```python
from build123d import *

# Parameters (mm, degrees)
BOSS_EXTRU_1_DEPTH      = 7.62
ESQUISSE3_W             = 0.8
ESQUISSE3_H             = 1.27
ENL_V_MAT_EXTRU_1_DEPTH = 8.9
ESQUISSE4_W             = 2.4
ESQUISSE4_H             = 0.5
ENL_V_MAT_EXTRU_2_DEPTH = 8.62
ESQUISSE2_W             = 0.6
ESQUISSE2_H             = 0.6
BOSS_EXTRU_2_DEPTH      = 3.5
BOSS_EXTRU_2_DEPTH_BACK = 9
BOSS_EXTRU_3_DEPTH      = 5.08
CHANFREIN4_SIZE         = 0.15
CHANFREIN5_SIZE         = 0.4


with BuildPart() as part:
    # Esquisse1 → Boss.-Extru.1 (new body)
    with BuildSketch(Plane.XY):
        Polygon((0, 11.4), (0, 0), (5, 0), (5, 11.4), (4.2, 11.4), (4.2, 2.5), (0.8, 2.5), (0.8, 11.4), align=None)
    extrude(amount=BOSS_EXTRU_1_DEPTH)

    # Esquisse3 → Enlèv. mat.-Extru.1 (cut)
    with BuildSketch(Plane(origin=(0, 11.4, 0), x_dir=(1, 0, 0), z_dir=(0, 1, 0))):
        with Locations((0.4, -0.635)):
            Rectangle(ESQUISSE3_W, ESQUISSE3_H)
        with Locations((0.4, -6.985)):
            Rectangle(ESQUISSE3_W, ESQUISSE3_H)
    extrude(amount=-ENL_V_MAT_EXTRU_1_DEPTH, mode=Mode.SUBTRACT)

    # Esquisse4 → Enlèv. mat.-Extru.2 (cut, through all)
    with BuildSketch(Plane.XY.offset(7.62)):
        with Locations((2.5, 0.25)):
            Rectangle(ESQUISSE4_W, ESQUISSE4_H)
    extrude(amount=-ENL_V_MAT_EXTRU_2_DEPTH, mode=Mode.SUBTRACT)

    # Esquisse2 → Boss.-Extru.2 (add, two sides)
    with BuildSketch(Plane.XZ.offset(-0.5)) as boss_extru_2_sk:
        with Locations((2.5, 6.35)):
            Rectangle(ESQUISSE2_W, ESQUISSE2_H)
        with Locations((2.5, 1.27)):
            Rectangle(ESQUISSE2_W, ESQUISSE2_H)
        with Locations((2.5, 3.81)):
            Rectangle(ESQUISSE2_W, ESQUISSE2_H)
    extrude(amount=BOSS_EXTRU_2_DEPTH)
    extrude(boss_extru_2_sk.sketch, amount=-BOSS_EXTRU_2_DEPTH_BACK)

    # Esquisse5 → Boss.-Extru.3 (add)
    with BuildSketch(Plane.XY.offset(6.35)):
        Polygon((0.8, 9.5), (1.2, 8.5), (0.8, 8.5), align=None)
    extrude(amount=-BOSS_EXTRU_3_DEPTH)

    # Chanfrein4
    chanfrein4_edges = [part.edges().sort_by_distance(p)[0] for p in [
        (2.8, 9.5, 3.81),
        (2.5, 9.5, 3.51),
        (2.2, 9.5, 3.81),
        (2.5, 9.5, 4.11),
        (2.8, -3, 3.81),
        (2.5, -3, 4.11),
        (2.2, -3, 3.81),
        (2.5, -3, 3.51),
        (2.8, 9.5, 6.35),
        (2.5, 9.5, 6.05),
        (2.2, 9.5, 6.35),
        (2.5, 9.5, 6.65),
        (2.8, -3, 6.35),
        (2.5, -3, 6.65),
        (2.2, -3, 6.35),
        (2.5, -3, 6.05),
        (2.8, 9.5, 1.27),
        (2.5, 9.5, 0.97),
        (2.2, 9.5, 1.27),
        (2.5, 9.5, 1.57),
        (2.8, -3, 1.27),
        (2.5, -3, 1.57),
        (2.2, -3, 1.27),
        (2.5, -3, 0.97),
    ]]
    chamfer(chanfrein4_edges, length=CHANFREIN4_SIZE)

    # Chanfrein5
    chanfrein5_edges = [part.edges().sort_by_distance(p)[0] for p in [
        (4.2, 11.4, 3.81),
        (0.8, 11.4, 3.81),
    ]]
    chamfer(chanfrein5_edges, length=CHANFREIN5_SIZE)


solid = part.part
```
The model under review builds one solid part; all positions refer to its coordinate system, in mm. A direction names the side the tool comes from. Round coordinates to 2 decimals unless told otherwise and drop trailing zeros. Order: outer loops, then holes, each group sorted by start corner. A loop starts at its lowest first (then second) coordinate and runs counter-clockwise, first axis right, second up. Notation, with made-up numbers: (7, 50) -> (66, 50) arc R19 ccw to (66, 87) -> close; hole circle Ø9 at (30.5, 66.5). An arc over 180 degrees is marked (long way). One line per item, written item: value. Start each with the question number.
Q1. Take a section at C-C (z = 4.5). Write out the cut boundary in (x, y), and give its area (3 significant figures).
Q2. Mouldability with a two-part tool opening along Y and no side actions: class faces 4 (the face through (1, 0, 4)), 5 (the face through (3, 2, 0)), 6 (the face through (1, 9, 4)), 7 (the face through (0.8, 5, 4)) as released by +Y, released by -Y, zero draft, split by the parting line, or undercut.
Q3. Machinability: for faces 1 (the face through (4, 0, 4)), 2 (the face through (0.5, 7, 6.35)), 3 (the face through (0.8, 10, 4)), which of the approach directions +Z, -Z, +X, -X, +Y, -Y give a long, thin tool a straight path to every point of the face, cutting with its end or side? Answer none if there is none.
Q4. Take a section at A-A (y = -0.25). Write out the cut boundary in (x, z).
Q5. Clearance check with flat-ended pins moving along their axes: pin 1 Ø1 at (x, y) = (2.5, 6.5) entering from -Z; pin 2 Ø0.5 at (y, z) = (-1.5, 4) entering from -X; pin 3 Ø2 at (x, y) = (1, 9) entering from -Z. State where each tip first meets the part, or that it passes through.
Q6. Take a section at B-B (y = 8). Write out the cut boundary in (x, z).
Q7. Wall thickness on line 1 (Z direction, x = 2.7, y = 6.75); line 2 (X direction, y = 7.25, z = 6); line 3 (X direction, y = 6.5, z = 0.5): over which ranges is each line inside the solid? List them lowest first.
Q8. Take a section at D-D (x = 1.85). Write out the cut boundary in (y, z).
Reported:
1. outline: (0, 0) -> (1.3, 0) -> (1.3, 0.5) -> (3.7, 0.5) -> (3.7, 0) -> (5, 0) -> (5, 11.4) -> (4.6, 11.4) -> (4.2, 11) -> (4.2, 2.5) -> (0.8, 2.5) -> (0.8, 8.5) -> (1.2, 8.5) -> (0.8, 9.5) -> (0.8, 11) -> (0.4, 11.4) -> (0, 11.4) -> close
1. area: 25.6 mm2
2. face 4: released by -Y
2. face 5: zero draft
2. face 6: released by +Y
2. face 7: undercut
3. face 1: +Z, -Z, +X, -Y
3. face 2: +Z, -X, +Y
3. face 3: +Z, -Z, +Y
4. outline: (2.2, 0.97) -> (2.8, 0.97) -> (2.8, 1.57) -> (2.2, 1.57) -> close; (2.2, 3.51) -> (2.8, 3.51) -> (2.8, 4.11) -> (2.2, 4.11) -> close; (2.2, 6.05) -> (2.8, 6.05) -> (2.8, 6.65) -> (2.2, 6.65) -> close
5. pin 1: stops at z = 0.97
5. pin 2: stops at x = 2.2
5. pin 3: stops at z = 1.27
6. outline: (0, 1.27) -> (0.8, 1.27) -> (0.8, 6.35) -> (0, 6.35) -> close; (2.2, 0.97) -> (2.8, 0.97) -> (2.8, 1.57) -> (2.2, 1.57) -> close; (2.2, 3.51) -> (2.8, 3.51) -> (2.8, 4.11) -> (2.2, 4.11) -> close; (2.2, 6.05) -> (2.8, 6.05) -> (2.8, 6.65) -> (2.2, 6.65) -> close; (4.2, 0) -> (5, 0) -> (5, 7.62) -> (4.2, 7.62) -> close
7. line 1: z = 0.97 to 1.57, 3.51 to 4.11, 6.05 to 6.65
7. line 2: x = 0 to 0.8, 4.2 to 5
7. line 3: x = 4.2 to 5
8. outline: (0.5, 0) -> (2.5, 0) -> (2.5, 7.62) -> (0.5, 7.62) -> close
